Geometry check sheet. Reference: the model listing, model coordinates, mm. Round coordinates to 2 decimals unless told otherwise and drop trailing zeros. Order: outer loops, then holes, each group sorted by start corner. A loop starts at its lowest first (then second) coordinate and runs counter-clockwise, first axis right, second up.
(1) Release check for a two-part mould opening along X. For faces 1 (the face through (-1, 0, -7.5)), 2 (the face through (44, 0, 0)), 3 (the face through (-44, 0, 0)), 4 (the face through (-0.54, 0.06, 2.44)) record: +X half, -X half, draft (parallel to the pull), parting line (faces both ways), or undercut.
(2) Sectioned sample at B-B (z = 0). Record the boundary of the cut face in (x, y), plus the area to 3 significant figures.
(3) Sectioned sample at A-A (x = 0). Record the boundary of the cut face in (y, z).
(4) Sectioned sample at C-C (y = -3). Record the boundary of the cut face in (x, z).
(5) Material ranges on line 1 along X through (y, z) = (-3.5, 1.25); line 2 along Z through (x, y) = (35, -1.25); line 3 along X through (y, z) = (-1.5, 0.75), recorded low to high.
from build123d import *

# Parameters (mm, degrees)
SKETCH_2_W         = 88
SKETCH_2_H         = 8
EXTRUDE_1_DEPTH    = 7.5
HOLE_WIZARD_M6_1_D = 5


with BuildPart() as part:
    # 草图2 → 凸台-拉伸1 (new, symmetric)
    with BuildSketch(Plane.XY):
        Rectangle(SKETCH_2_W, SKETCH_2_H)
    extrude(amount=EXTRUDE_1_DEPTH, both=True)

    # M6 螺纹孔1 (through all)
    with Locations(Plane(origin=(0, -4, 0), x_dir=(-1, 0, 0), z_dir=(0, -1, 0))):
        with Locations((35, 0), (-35, 0), (0, 0)):
            Hole(HOLE_WIZARD_M6_1_D / 2)


solid = part.part
Answer below:
1. face 1: draft
1. face 2: +X half
1. face 3: -X half
1. face 4: undercut
2. outline: (-44, -4) - (-37.5, -4) - (-37.5, 4) - (-44, 4) - close; (-32.5, -4) - (-2.5, -4) - (-2.5, 4) - (-32.5, 4) - close; (2.5, -4) - (32.5, -4) - (32.5, 4) - (2.5, 4) - close; (37.5, -4) - (44, -4) - (44, 4) - (37.5, 4) - close
2. area: 584 mm2
3. outline: (-4, -7.5) - (4, -7.5) - (4, -2.5) - (-4, -2.5) - close; (-4, 2.5) - (4, 2.5) - (4, 7.5) - (-4, 7.5) - close
4. outline: (-44, -7.5) - (44, -7.5) - (44, 7.5) - (-44, 7.5) - close; hole circle Ø5 at (-35, 0); hole circle Ø5 at (0, 0); hole circle Ø5 at (35, 0)
5. line 1: x = -44 to -37.17, -32.83 to -2.17, 2.17 to 32.83, 37.17 to 44
5. line 2: z = -7.5 to -2.5, 2.5 to 7.5
5. line 3: x = -44 to -37.38, -32.62 to -2.38, 2.38 to 32.62, 37.38 to 44
